Read the model definition and answer for the solid it produces. Units are mm, in the model's axes. A direction names the side the tool comes from. Coordinates: 2 decimals unless noted, no trailing zeros. Write each loop counter-clockwise with the first axis right and the second up, starting at its lowest first coordinate (ties: lowest second). Pieces come first, ordered by that corner, then holes. Notation, with made-up numbers: (-2.75, 74.5) -> (17.25, 74.5) arc R18 ccw to (17.25, 98.5) -> close; hole circle Ø1 at (56, 49.25). An arc over 180 degrees is marked (long way). Write item = value, one per line. Start each with the question number.
1) For a pull along Y with two mould halves and no side action, classify faces 1 (the face through (-4, 0, -63)), 2 (the face through (-22, 21, -127)), 3 (the face through (-31.75, 17, -9)) as released by +Y, released by -Y, zero draft, split by the parting line, or undercut.
2) Find the intervals of material crossed by line 1 along X through (y, z) = (4.25, -120.65) (3 decimals); line 2 along Z through (x, y) = (-44.45, 10) (3 decimals); line 3 along Z through (x, y) = (37.5, 67), in increasing order. Write a range as from..to.
3) A tool of negligible diameter and unlimited length cuts with its end or side. For faces 4 (the face through (35, 44, -35.3)), 5 (the face through (28.956, 44, -57)), 6 (the face through (-19.05, 17, -9)), from which of +Z, -Z, +X, -X, +Y, -Y can it reach the whole face along a straight path? Write none if from no direction.
4) Section B-B (y = 54) is taken. Determine the outline of the cut face in (x, z).
5) Section C-C (x = -16) is taken. Determine the outline of the cut face in (y, z).
6) Section A-A (x = -44.45) is taken. Determine the outline of the cut face in (y, z) (3 decimals), plus the area to 3 significant figures.
7) Flat-ended cylindrical pins translate along their axes: pin 1 Ø5 at (x, z) = (-15, -5.5) entering from -Y; pin 2 Ø16.5 at (y, z) = (44.45, -12.67) entering from -X; pin 3 Ø7.5 at (y, z) = (44.45, -63.47) entering from +X; pin 4 Ø2 at (x, z) = (-2, -40) entering from +Y. Find the tip coordinate at first contact, or state that the pin passes through.
8) Section D-D (x = 33) is taken. Determine the outline of the cut face in (y, z).
Autodesk Inventor part; units mm, degrees
ref_plane "YZ Plane" through (0, 0, 0) normal (1, 0, 0) x (0, 1, 0)
ref_plane "XZ Plane" through (0, 0, 0) normal (0, 1, 0) x (-1, 0, 0)
ref_plane "XY Plane" through (0, 0, 0) normal (0, 0, 1) x (1, 0, 0)
sketch "Sketch1" plane through (0, 0, 0) normal (0, 1, 0) x (-1, 0, 0)
  line L0 (3.175, 0) -> (47.625, 0)
  line L1 (50.8, -3.175) -> (50.8, -123.825)
  line L2 (47.625, -127) -> (3.175, -127)
  arc A0 (50.8, -3.175) -> (47.625, 0) centre (47.625, -3.175) ccw
  arc A1 (47.625, -127) -> (50.8, -123.825) centre (47.625, -123.825) ccw
  line L3 (0, 0) -> (-41.656, 0)
  line L4 (-41.656, 0) -> (-41.656, -127)
  line L5 (-41.656, -127) -> (0, -127)
  line L6 (3.175, -127) -> (0, -127)
  line L7 (3.175, 0) -> (0, 0)
  point P0 (50.8, -127)
  point P1 (50.8, 0)
  point P2 (0, -127)
  dimension "d0" = 50.8
  dimension "d1" = 127
  dimension "d4" = 3.175
  dimension "d39" = 41.656
  dimension "d40" = 127
extrude "Extrusion1" add sketch "Sketch1" along normal blind 12.7
sketch "Sketch2" plane through (0, 12.7, 0) normal (0, 1, 0) x (1, 0, 0)
  line L0 (0, 0) -> (-6.35, 0) construction
  line L1 (-6.35, 0) -> (-6.35, 6.35) construction
  line L2 (-6.35, 6.35) -> (0, 6.35) construction
  line L3 (0, 6.35) -> (0, 0) construction
  circle A0 centre (-6.35, 6.35) radius 3.175
  line L4 (0, 3.175) -> (0, 123.825) construction
  line L5 (0, 63.5) -> (-50.8802, 63.5) construction
  line L6 (-50.8802, 63.5) -> (-25.4, 127) construction
  line L7 (41.656, 127) -> (-47.625, 127) construction
  line L8 (-25.4, 127) -> (-25.4, 0) construction
  line L9 (-47.625, 0) -> (41.656, 0) construction
  circle A1 centre (-6.35, 120.65) radius 3.175
  circle A2 centre (-44.45, 6.35) radius 3.175
  circle A3 centre (-44.45, 120.65) radius 3.175
  point P0 (-3.175, 127)
  point P1 (-3.175, 0)
  dimension "d5" = 6.35
  dimension "d6" = 6.35
  dimension "d7" = 6.35
extrude "Extrusion2" cut sketch "Sketch2" against normal through all
sketch "Sketch3" plane through (0, 12.7, 0) normal (0, 1, 0) x (1, 0, 0)
  line L0 (0, 0) -> (-12.7, 0) construction
  line L1 (0, 0) -> (12.7, 0) construction
  line L2 (-47.625, 0) -> (41.656, 0) construction
  line L3 (-25.4, 0) -> (-25.4, 127) construction
  line L4 (41.656, 127) -> (-47.625, 127) construction
  line L5 (-50.8, 0) -> (-38.1, 0) construction
  line L6 (-38.1, 0) -> (-12.7, 0)
  line L7 (-12.7, 0) -> (-12.7, 127)
  line L8 (-12.7, 127) -> (-38.1, 127)
  line L9 (-38.1, 127) -> (-38.1, 0)
  point P0 (-3.175, 0)
  point P1 (-3.175, 127)
  dimension "d14" = 12.7
  dimension "d15" = 180
  dimension "d36" = 25.4
extrude "Extrusion3" add sketch "Sketch3" along normal blind 63.5
sketch "Sketch5" plane through (-12.7, 12.7, 0) normal (1, 0, 0) x (0, 0, -1)
  line L0 (0, 63.5) -> (127, 63.5) construction
  line L1 (63.5, 63.5) -> (63.5, 0) construction
  line L2 (123.825, 0) -> (3.175, 0) construction
  line L3 (127, 0) -> (127, 63.5) construction
  circle A0 centre (63.4683, 31.7498) radius 6.35
  circle A1 centre (12.6683, 31.7498) radius 6.35
  circle A2 centre (114.2683, 31.7498) radius 6.35
  line L4 (0, 0) -> (0, 63.5) construction
  line L5 (0, 31.75) -> (127, 31.75) construction
  point P0 (0, -12.7)
  dimension "d24" = 12.7
  dimension "d27" = 12.7
  dimension "d37" = 50.8
  dimension "d38" = 50.8
extrude "Extrusion5" cut sketch "Sketch5" against normal through all
sketch "Sketch6" plane through (0, 12.7, 0) normal (0, 1, 0) x (1, 0, 0)
  line L0 (-12.7, 0) -> (-19.05, 0)
  line L1 (-19.05, 0) -> (-19.05, 19.05)
  line L2 (-19.05, 19.05) -> (-12.7, 19.05)
  line L3 (-12.7, 19.05) -> (-12.7, 0)
  line L4 (-38.1, 127) -> (-38.1, 0) construction
  line L5 (-38.4604, 63.7403) -> (-13.0604, 63.7086) construction
  line L6 (-12.7, 69.8183) -> (-12.7, 57.1183) construction
  line L7 (-12.541, 127.416) -> (-18.891, 127.4319)
  line L8 (-18.891, 127.4319) -> (-18.9385, 108.3819)
  line L9 (-18.9385, 108.3819) -> (-12.5885, 108.3661)
  line L10 (-12.5885, 108.3661) -> (-12.541, 127.416)
  line L11 (-47.625, 0) -> (41.656, 0) construction
  line L12 (-25.4, 0) -> (-25.4, 127) construction
  line L13 (41.656, 127) -> (-47.625, 127) construction
  line L14 (-38.1, 0) -> (-31.75, 0)
  line L15 (-31.75, 0) -> (-31.75, 19.05)
  line L16 (-31.75, 19.05) -> (-38.1, 19.05)
  line L17 (-38.1, 19.05) -> (-38.1, 0)
  line L18 (-38.1, 69.8183) -> (-38.1, 57.1183) construction
  line L19 (-38.259, 127.416) -> (-31.909, 127.4319)
  line L20 (-31.909, 127.4319) -> (-31.8615, 108.3819)
  line L21 (-31.8615, 108.3819) -> (-38.2115, 108.3661)
  line L22 (-38.2115, 108.3661) -> (-38.259, 127.416)
  line L23 (-47.625, 0) -> (-2.456, 0) construction
  point P0 (0, 0)
  point P1 (-3.175, 0)
  point P2 (-3.175, 127)
  point P3 (-37.7396, 63.7086)
  point P4 (-38.1, 69.8183)
  point P5 (-38.1, 57.1183)
  dimension "d30" = 6.35
  dimension "d31" = 19.05
extrude "Extrusion6" cut sketch "Sketch6" along normal blind 8.382
sketch "Sketch7" plane through (0, 12.7, 0) normal (0, 1, 0) x (1, 0, 0)
  line L0 (41.5616, 127.6536) -> (41.5616, 0) construction
  line L1 (41.656, 0) -> (41.656, 127)
  line L2 (41.656, 63.5) -> (28.956, 63.5) construction
  line L3 (28.956, 63.5) -> (28.956, 35.3)
  line L4 (28.956, 35.3) -> (41.656, 35.3)
  line L5 (41.656, 35.3) -> (41.656, 63.5)
  line L6 (28.956, 63.5) -> (28.956, 91.7)
  line L7 (28.956, 91.7) -> (41.656, 91.7)
  line L8 (41.656, 91.7) -> (41.656, 63.5)
  point P0 (0, 0)
  dimension "d41" = 12.7
  dimension "d42" = 28.2
extrude "Extrusion7" add sketch "Sketch7" along normal blind 63.5
sketch "Sketch8" plane through (41.656, 0, 0) normal (1, 0, 0) x (0, 0, -1)
  line L0 (127, 0) -> (123.825, 0) construction
  line L1 (0, 0) -> (127, 0) construction
  line L2 (123.825, 0) -> (3.175, 0) construction
  line L3 (63.5, 0) -> (63.5, 13.8176) construction
  circle A0 centre (63.4683, 44.4498) radius 6.35 construction
  line L4 (63.5, 13.8176) -> (63.4683, 44.4498) construction
  circle A1 centre (63.4683, 44.4498) radius 19.05
  dimension "d45" = 13.8176
  dimension "d46" = 38.1
extrude "Extrusion8" cut sketch "Sketch8" against normal blind 1.6
sketch "Sketch9" plane through (41.656, 0, 0) normal (1, 0, 0) x (0, 0, -1)
  line L0 (127, 0) -> (123.825, 0) construction
  line L1 (0, 0) -> (127, 0) construction
  line L2 (123.825, 0) -> (3.175, 0) construction
  line L3 (63.5, 0) -> (63.5, 13.8176) construction
  circle A0 centre (63.4683, 44.4498) radius 3.25
  line L4 (63.5, 13.8176) -> (63.4683, 44.4498) construction
  circle A1 centre (63.4683, 44.4498) radius 19.05 construction
  dimension "d49" = 13.8176
  dimension "d50" = 38.1
  dimension "d51" = 6.5
extrude "Extrusion9" cut sketch "Sketch9" against normal through all
sketch "Sketch10" plane through (41.656, 0, 0) normal (1, 0, 0) x (0, 0, -1)
  line L0 (127, 0) -> (123.825, 0) construction
  line L1 (0, 0) -> (127, 0) construction
  line L2 (123.825, 0) -> (3.175, 0) construction
  line L3 (63.5, 0) -> (63.5, 13.8176) construction
  circle A0 centre (63.4683, 44.4498) radius 6.35 construction
  line L4 (63.5, 13.8176) -> (63.4683, 44.4498) construction
  circle A1 centre (63.4683, 44.4498) radius 19.05 construction
  line L5 (87.0383, 68.0198) -> (39.8983, 68.0198) construction
  line L6 (39.8983, 68.0198) -> (39.8983, 20.8798) construction
  line L7 (39.8983, 20.8798) -> (87.0383, 20.8798) construction
  line L8 (87.0383, 20.8798) -> (87.0383, 68.0198) construction
  circle A2 centre (63.4683, 44.4498) radius 3.25 construction
  line L9 (87.0383, 68.0198) -> (39.8983, 20.8798) construction
  line L10 (39.8983, 68.0198) -> (87.0383, 20.8798) construction
  circle A3 centre (87.0383, 20.8798) radius 2.5
  circle A4 centre (39.8984, 20.8798) radius 2.5
  circle A5 centre (39.8983, 68.0198) radius 2.5
  circle A6 centre (87.0383, 68.0198) radius 2.5
  dimension "d54" = 13.8176
  dimension "d55" = 38.1
  dimension "d56" = 47.14
  dimension "d57" = 47.14
  dimension "d58" = 5
  dimension "d59" = 5
  dimension "d60" = 5
  dimension "d61" = 5
extrude "Extrusion10" cut sketch "Sketch10" against normal up to surface (12.7 mm away)
sketch "Sketch11" plane through (0, 0, 0) normal (0, -1, 0) x (1, 0, 0)
  line L0 (41.656, 0) -> (41.656, -35.3) construction
  line L1 (41.656, 0) -> (-47.625, 0) construction
  line L2 (-50.8, -3.175) -> (-50.8, -123.825) construction
  line L3 (-47.625, -127) -> (41.656, -127) construction
  line L4 (41.656, -127) -> (41.656, 0) construction
  arc A0 (-47.625, 0) -> (-50.8, -3.175) centre (-47.625, -3.175) ccw construction
  arc A1 (-50.8, -123.825) -> (-47.625, -127) centre (-47.625, -123.825) ccw construction
  circle A2 centre (-44.45, -6.35) radius 3.175 construction
  circle A3 centre (-44.45, -6.35) radius 3.175 construction
  circle A4 centre (-6.35, -6.35) radius 3.175 construction
  circle A5 centre (-6.35, -6.35) radius 3.175 construction
  circle A6 centre (-44.45, -120.65) radius 3.175 construction
  circle A7 centre (-44.45, -120.65) radius 3.175 construction
  circle A8 centre (-6.35, -120.65) radius 3.175 construction
  circle A9 centre (-6.35, -120.65) radius 3.175 construction
  point P0 (0, 0)
  dimension "d64" = 3.175
properties part number "Near Gantry Bracket"
Answer key:
q1.face_1 = released by -Y
q1.face_2 = zero draft
q1.face_3 = undercut
q2.line_1 = -50.8..-47.625, -41.275..-9.525, -3.175..41.656
q2.line_2 = -127..-123.825, -117.475..-9.525, -3.175..0
q2.line_3 = -91.7..-89.32, -84.76..-42.18, -37.62..-35.3
q3.face_4 = +Z, +X, +Y
q3.face_5 = +Z, -Z, +Y
q3.face_6 = +Z, +X
q4.outline = (-38.1, -127) -> (-12.7, -127) -> (-12.7, 0) -> (-38.1, 0) -> close; (28.96, -91.7) -> (41.66, -91.7) -> (41.66, -79.95) -> (40.06, -79.95) -> (40.06, -46.99) -> (41.66, -46.99) -> (41.66, -35.3) -> (28.96, -35.3) -> close
q5.outline = (0, -127) -> (12.7, -127) -> (12.7, -108.37) -> (21.08, -108.37) -> (21.08, -127) -> (76.2, -127) -> (76.2, 0) -> (21.08, 0) -> (21.08, -19.05) -> (12.7, -19.05) -> (12.7, 0) -> (0, 0) -> close; hole circle Ø12.7 at (44.45, -114.27); hole circle Ø12.7 at (44.45, -63.47); hole circle Ø12.7 at (44.45, -12.67)
q6.outline = (0, -127) -> (12.7, -127) -> (12.7, -123.825) -> (0, -123.825) -> close; (0, -117.475) -> (12.7, -117.475) -> (12.7, -9.525) -> (0, -9.525) -> close; (0, -3.175) -> (12.7, -3.175) -> (12.7, 0) -> (0, 0) -> close
q6.area = 1,450 mm^2
q7.pin_1 = 0
q7.pin_2 = -38.1
q7.pin_3 = 40.06
q7.pin_4 = 12.7
q8.outline = (0, -127) -> (12.7, -127) -> (12.7, -91.7) -> (76.2, -91.7) -> (76.2, -35.3) -> (12.7, -35.3) -> (12.7, 0) -> (0, 0) -> close; hole circle Ø5 at (20.88, -87.04); hole circle Ø5 at (20.88, -39.9); hole circle Ø6.5 at (44.45, -63.47); hole circle Ø5 at (68.02, -87.04); hole circle Ø5 at (68.02, -39.9)
